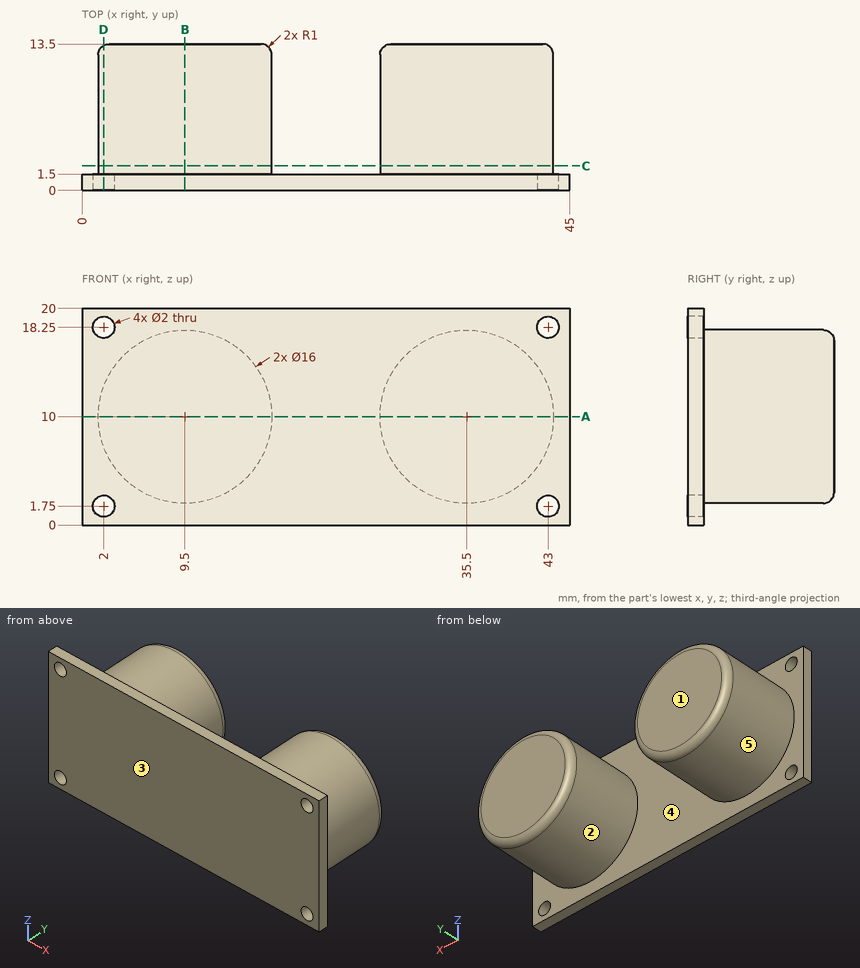
The drawing under review shows one solid part. Ordinate dimensions are in mm from its lowest x, y, z. A direction names the side the tool comes from. Give positions to 0.01 mm unless a question says otherwise; leave off trailing zeros. Write each loop counter-clockwise with the first axis right and the second up, starting at its lowest first coordinate (ties: lowest second). Pieces come first, ordered by that corner, then holes.
1. For P1, Ø2, axis at x = 30, y = 6, coming from the +Z side; P2, Ø2, axis at x = 18.5, z = 16, coming from the +Y side; P3, Ø2, axis at y = 7.5, z = 3, coming from the +X side, all flat-tipped, find the tip position at first contact; note any pin that passes through.
2. Add section B-B, the plane x = 9.5. Write out the cut boundary in (y, z).
3. Add section C-C, the plane y = 2.25. Write out the cut boundary in (x, z), plus the area to 3 significant figures.
4. Wall thickness on L1, parallel to X at y = 0.8, z = 1.75; L2, parallel to Z at x = 2, y = 0.75; L3, parallel to Y at x = 18, z = 17.25: over which ranges is each line inside the solid? List them lowest first.
5. Add section D-D, the plane x = 2. Count the separate pieces of the cut face and the enclosed holes in it, plus the area to 3 significant figures.
6. Draft analysis for pull direction X (two halves, no side actions). For the marked faces 3, 4 and 5, state which applies: +X half, -X half, draft (parallel to the pull), parting line (faces both ways), or undercut.
7. Add section A-A, the plane z = 10. Write out the cut boundary in (x, y), plus the area to 3 significant figures.
8. Tool access review of the marked faces 1 and 2: name each direction out of +Z, -Z, +X, -X, +Y, -Y from which nothing blocks a thin tool from reaching the whole face with its end or side.
Worked answers:
1. P1: stops at z = 16.61
1. P2: stops at y = 1.5
1. P3: stops at x = 40.79
2. outline: (0, 0) - (1.5, 0) - (1.5, 2) - (12.5, 2) arc R1 ccw to (13.5, 3) - (13.5, 17) arc R1 ccw to (12.5, 18) - (1.5, 18) - (1.5, 20) - (0, 20) - close
3. outline: circle Ø16 at (9.5, 10); circle Ø16 at (35.5, 10)
3. area: 402 mm2
4. L1: x = 0 to 1, 3 to 42, 44 to 45
4. L2: z = 0 to 0.75, 2.75 to 17.25, 19.25 to 20
4. L3: y = 0 to 1.5
5. separate pieces: 3
5. enclosed holes: 0
5. area: 89.2 mm2
6. face 3: draft
6. face 4: undercut
6. face 5: undercut
7. outline: (0, 0) - (45, 0) - (45, 1.5) - (43.5, 1.5) - (43.5, 12.5) arc R1 ccw to (42.5, 13.5) - (28.5, 13.5) arc R1 ccw to (27.5, 12.5) - (27.5, 1.5) - (17.5, 1.5) - (17.5, 12.5) arc R1 ccw to (16.5, 13.5) - (2.5, 13.5) arc R1 ccw to (1.5, 12.5) - (1.5, 1.5) - (0, 1.5) - close
7. area: 451 mm2
8. face 1: +Z, -Z, +X, -X, +Y
8. face 2: +Y
